Can you work these out from the drawing? Everything is in mm from the part's minimum corner. Give positions to 0.01 mm unless a question says otherwise; leave off trailing zeros.
Q1. Will this pin go through, and if not, where does the flat tip stop? P1, Ø6.5, axis at x = 140, y = 108.5, coming from the +Z side.
Q2. We'd pull the mould along Z, two halves only. Please class the marked faces 1, 2 and 3: +Z half, -Z half, draft (parallel to the pull), parting line (faces both ways), or undercut.
Q3. I need wall thicknesses on line 1 (Y direction, x = 139.7, z = 112); line 2 (X direction, y = 111, z = 93); line 3 (Z direction, x = 138, y = 382.5). Which ranges of each line are inside material? Lowest first, please.
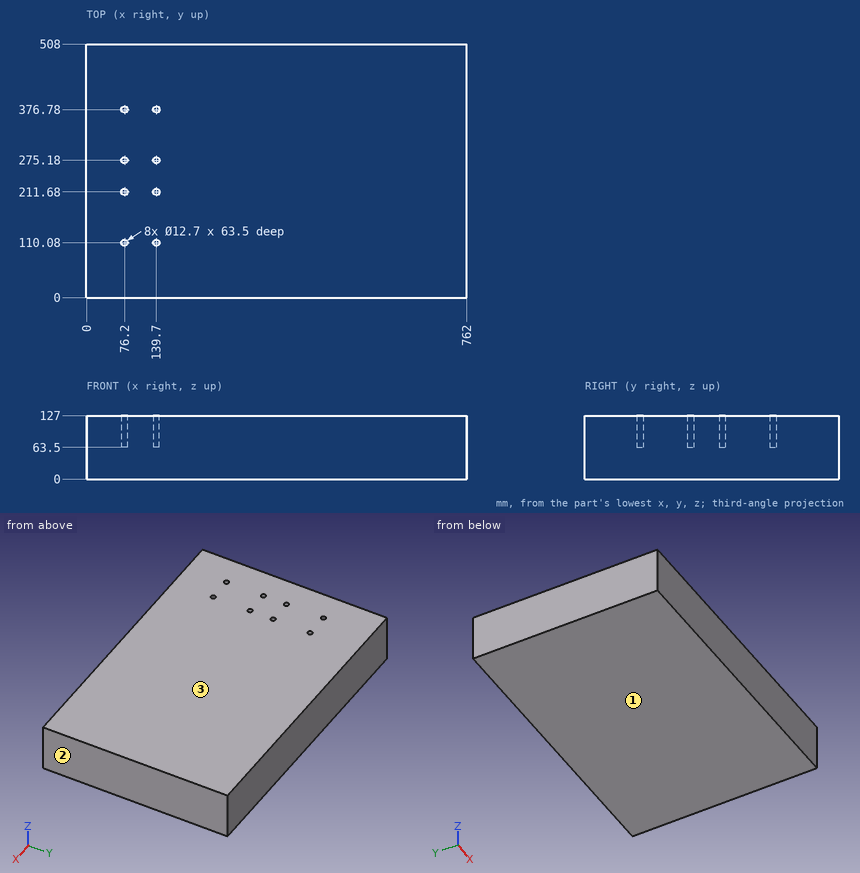
Check sheet entries:
1. P1: stops at z = 63.5
2. face 1: -Z half
2. face 2: draft
2. face 3: +Z half
3. line 1: y = 0 to 103.73, 116.43 to 205.33, 218.03 to 268.83, 281.53 to 370.43, 383.13 to 508
3. line 2: x = 0 to 69.92, 82.48 to 133.42, 145.98 to 762
3. line 3: z = 0 to 63.5
